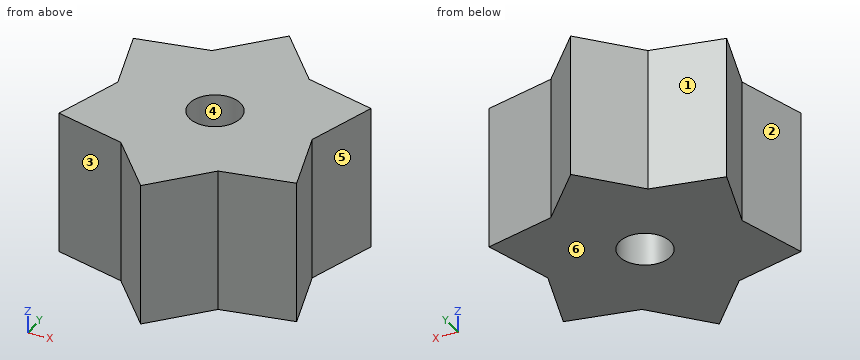
```python
from build123d import *

# Parameters (mm, degrees)
SKETCH1_R           = 1.15
BOSS_EXTRUDE1_DEPTH = 6.5


with BuildPart() as part:
    # Sketch1 → Boss-Extrude1 (new body)
    with BuildSketch(Plane.XY):
        Polygon((0, -6.142777017), (2.175697935, -3.768419365), (5.319800946, -3.071388508), (4.351395869, 0), (5.319800946, 3.071388508), (2.175697935, 3.768419365), (0, 6.142777017), (-2.175697935, 3.768419365), (-5.319800946, 3.071388508), (-4.351395869, 0), (-5.319800946, -3.071388508), (-2.175697935, -3.768419365), align=None)
        Circle(SKETCH1_R, mode=Mode.SUBTRACT)
    extrude(amount=-BOSS_EXTRUDE1_DEPTH)


solid = part.part
```
Verification items for the finished model (mm, model axes). Face numbers are marked on the shaded views. A direction names the side the tool comes from. Give positions to 0.01 mm unless a question says otherwise; leave off trailing zeros. Order: outer loops, then holes, each group sorted by start corner. A loop starts at its lowest first (then second) coordinate and runs counter-clockwise, first axis right, second up. Notation, with made-up numbers: (16.5, 37) - (65.5, 37) arc R18 cw to (65.5, 57) - close; hole circle Ø4 at (43, 52). An arc over 180 degrees is marked (long way). Answer as CSV lines item,"result". Start each with the question number.
Item 1: Section check C-C, the plane x = -0.5. Record the boundary of the cut face in (y, z).
Item 2: Material ranges on L1, parallel to Y at x = -1, z = -3.25; L2, parallel to Y at x = -0.75, z = -5.25; L3, parallel to X at y = 0.5, z = -5, recorded low to high.
Item 3: Section check D-D, the plane x = 3. Record the boundary of the cut face in (y, z).
Item 4: Gauge pin test, flat ends, axial feed: pin 1 (2 mm diameter, centred on y = -2, z = -2.5, fed in from +X); pin 2 (1 mm diameter, centred on x = -3.5, z = -2, fed in from -Y). Record the tip position at first contact, or that the pin passes through.
Item 5: Section check A-A, the plane z = -4.5. Record the boundary of the cut face in (x, y), plus the area to 3 significant figures.
Item 6: Mould release check, pull along Y, two halves, no side actions. Record for the marked faces 3, 4, 5 and 6: released by +Y, released by -Y, zero draft, split by the parting line, or undercut.
Item 7: Access from +Z, -Z, +X, -X, +Y, -Y to the whole of each face (thin tool, end or side, straight path). Record for the marked faces 1 and 2.
Item 8: Section check B-B, the plane y = -0.5. Record the boundary of the cut face in (x, z), plus the area to 3 significant figures.
Filled in:
1,outline,"(-5.6, -6.5) - (-1.04, -6.5) - (-1.04, 0) - (-5.6, 0) - close; (1.04, -6.5) - (5.6, -6.5) - (5.6, 0) - (1.04, 0) - close"
2,L1,"-5.05 to -0.57, 0.57 to 5.05"
2,L2,"-5.32 to -0.87, 0.87 to 5.32"
2,L3,"-4.51 to -1.04, 1.04 to 4.51"
3,outline,"(-3.59, -6.5) - (3.59, -6.5) - (3.59, 0) - (-3.59, 0) - close"
4,pin 1,"x = 5.3"
4,pin 2,"y = -3.59"
5,outline,"(-5.32, -3.07) - (-2.18, -3.77) - (0, -6.14) - (2.18, -3.77) - (5.32, -3.07) - (4.35, 0) - (5.32, 3.07) - (2.18, 3.77) - (0, 6.14) - (-2.18, 3.77) - (-5.32, 3.07) - (-4.35, 0) - close; hole circle Ø2.3 at (0, 0)"
5,area,"76.0 mm^2"
6,face 3,"released by -Y"
6,face 4,"undercut"
6,face 5,"undercut"
6,face 6,"zero draft"
7,face 1,"+Z, -Z, -X, +Y"
7,face 2,"+Z, -Z, -X"
8,outline,"(-4.51, -6.5) - (-1.04, -6.5) - (-1.04, 0) - (-4.51, 0) - close; (1.04, -6.5) - (4.51, -6.5) - (4.51, 0) - (1.04, 0) - close"
8,area,"45.2 mm^2"
